Verification items for the finished model (mm, model axes). Face numbers are marked on the shaded views. A direction names the side the tool comes from. Round coordinates to 2 decimals unless told otherwise and drop trailing zeros. Write each loop counter-clockwise with the first axis right and the second up, starting at its lowest first coordinate (ties: lowest second). Pieces come first, ordered by that corner, then holes. Notation, with made-up numbers: (65.25, -35) -> (123.25, -35) arc R6 cw to (123.25, -24) -> close; hole circle Ø9 at (80.25, -14.75). An arc over 180 degrees is marked (long way). Answer as a JSON object with one key per item and string values. Group by question number.
(1) Sectioned sample at B-B on x = -26. Record the cut outline in (y, z).
(2) Gauge pin test, flat ends, axial feed: pin 1 Ø3 at (x, y) = (39.4, -17.4) entering from +Z; pin 2 Ø1.6 at (y, z) = (-19, 5) entering from -X; pin 3 Ø2.5 at (x, y) = (39.4, 17.4) entering from -Z. Record the tip position at first contact, or that the pin passes through.
(3) Sectioned sample at C-C on y = -9. Record the cut outline in (x, z).
(4) Sectioned sample at A-A on x = 39.4. Record the cut outline in (y, z), and give its area (3 significant figures).
(5) Sectioned sample at D-D on z = 3.25. Record the cut outline in (x, y).
(6) Scan lines: L1, parallel to Y at x = -39.4, z = 1.2; L2, parallel to Y at x = -25.5, z = 3.5; L3, parallel to Z at x = -5.5, y = 2. Record each from-to range of solid material in increasing order. Write a range as from..to.
(7) Set-up check for the marked faces 1 and 2: record each of +Z, -Z, +X, -X, +Y, -Y from which the full face is reachable in a straight line by a thin tool's end or side.
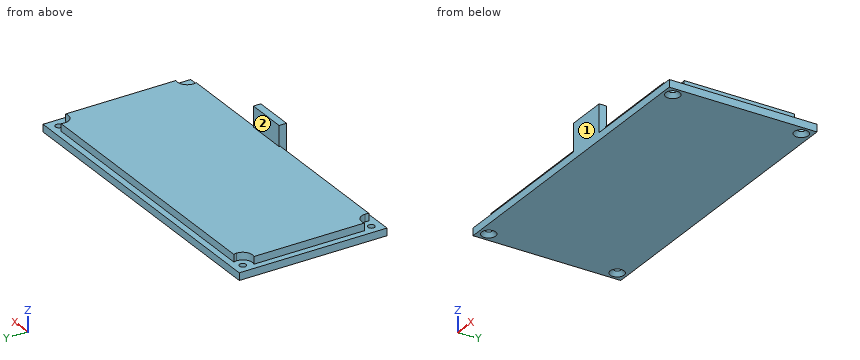
```python
from build123d import *

# Parameters (mm, degrees)
F0_W     = 84
F0_H     = 40
F1_DEPTH = 2
F3_DEPTH = 2
F4_R     = 0.9
F6_DEPTH = 2.001
F7_SIZE  = 1
F5_W     = 11
F5_H     = 7.5
F8_DEPTH = 2


with BuildPart() as f1:
    # F0 (on Top) → F1 (new body)
    with BuildSketch(Plane.XY):
        Rectangle(F0_W, F0_H)
    extrude(amount=F1_DEPTH)

    # F2 (on face) → F3 (join)
    with BuildSketch(Plane.XY.offset(2)):
        with BuildLine():
            Line((-36.9607378165, -18.3), (36.9607378165, -18.3))
            ThreePointArc((36.9607378165, -18.3), (37.5615223689, -15.5615223689), (40.3, -14.9607378165))
            Line((40.3, -14.9607378165), (40.3, 14.9607378165))
            ThreePointArc((40.3, 14.9607378165), (37.5615223689, 15.5615223689), (36.9607378165, 18.3))
            Line((36.9607378165, 18.3), (-36.9607378165, 18.3))
            ThreePointArc((-36.9607378165, 18.3), (-36.840499885, 17.8571205108), (-36.8, 17.4))
            ThreePointArc((-36.8, 17.4), (-37.9133931253, 15.2669270992), (-40.3, 14.9607378165))
            Line((-40.3, 14.9607378165), (-40.3, -14.9607378165))
            ThreePointArc((-40.3, -14.9607378165), (-37.9133931253, -15.2669270992), (-36.8, -17.4))
            ThreePointArc((-36.8, -17.4), (-36.840499885, -17.8571205108), (-36.9607378165, -18.3))
        make_face()
    extrude(amount=F3_DEPTH)

    # F4 (on face) → F6 (cut, through all)
    with BuildSketch(Plane.XY.offset(2)):
        with Locations((-39.4, 17.4)):
            Circle(F4_R)
        with Locations((-39.4, -17.4)):
            Circle(F4_R)
        with Locations((39.4, -17.4)):
            Circle(F4_R)
        with Locations((39.4, 17.4)):
            Circle(F4_R)
    extrude(amount=-F6_DEPTH, mode=Mode.SUBTRACT)

    # F7
    f7_edges = [f1.edges().sort_by_distance(p)[0] for p in [
        (-40.3, 17.4, 0),
        (-40.3, -17.4, 0),
        (38.5, -17.4, 0),
        (38.5, 17.4, 0),
    ]]
    chamfer(f7_edges, length=F7_SIZE)

    # F5 (on face) → F8 (join)
    with BuildSketch(Plane.XZ.offset(20)):
        with Locations((6.5, 5.75)):
            Rectangle(F5_W, F5_H)
    extrude(amount=-F8_DEPTH)


solid = f1.part
```
Computed values:
{
 "1": {"outline": "(-20, 0) -> (20, 0) -> (20, 2) -> (18.3, 2) -> (18.3, 4) -> (-18.3, 4) -> (-18.3, 2) -> (-20, 2) -> close"},
 "2": {"pin 1": "z = 2", "pin 2": "x = 1", "pin 3": "z = 0.65"},
 "3": {"outline": "(-42, 0) -> (42, 0) -> (42, 2) -> (40.3, 2) -> (40.3, 4) -> (-40.3, 4) -> (-40.3, 2) -> (-42, 2) -> close"},
 "4": {"outline": "(-20, 0) -> (-19.3, 0) -> (-18.3, 1) -> (-18.3, 2) -> (-20, 2) -> close; (-16.5, 1) -> (-15.5, 0) -> (15.5, 0) -> (16.5, 1) -> (16.5, 2) -> (14.8, 2) -> (14.8, 4) -> (-14.8, 4) -> (-14.8, 2) -> (-16.5, 2) -> close; (18.3, 1) -> (19.3, 0) -> (20, 0) -> (20, 2) -> (18.3, 2) -> close", "area": "130 mm2"},
 "5": {"outline": "(-40.3, -14.96) arc R2.6 cw to (-36.96, -18.3) -> (1, -18.3) -> (1, -20) -> (12, -20) -> (12, -18.3) -> (36.96, -18.3) arc R2.6 cw to (40.3, -14.96) -> (40.3, 14.96) arc R2.6 cw to (36.96, 18.3) -> (-36.96, 18.3) arc R2.6 cw to (-40.3, 14.96) -> close"},
 "6": {"L1": "-20..-18.3, -16.5..16.5, 18.3..20", "L2": "-18.3..18.3", "L3": "0..4"},
 "7": {"face 1": "+Z, -Z, +X, -X, -Y", "face 2": "+Z, +X, -X, +Y"}
}
